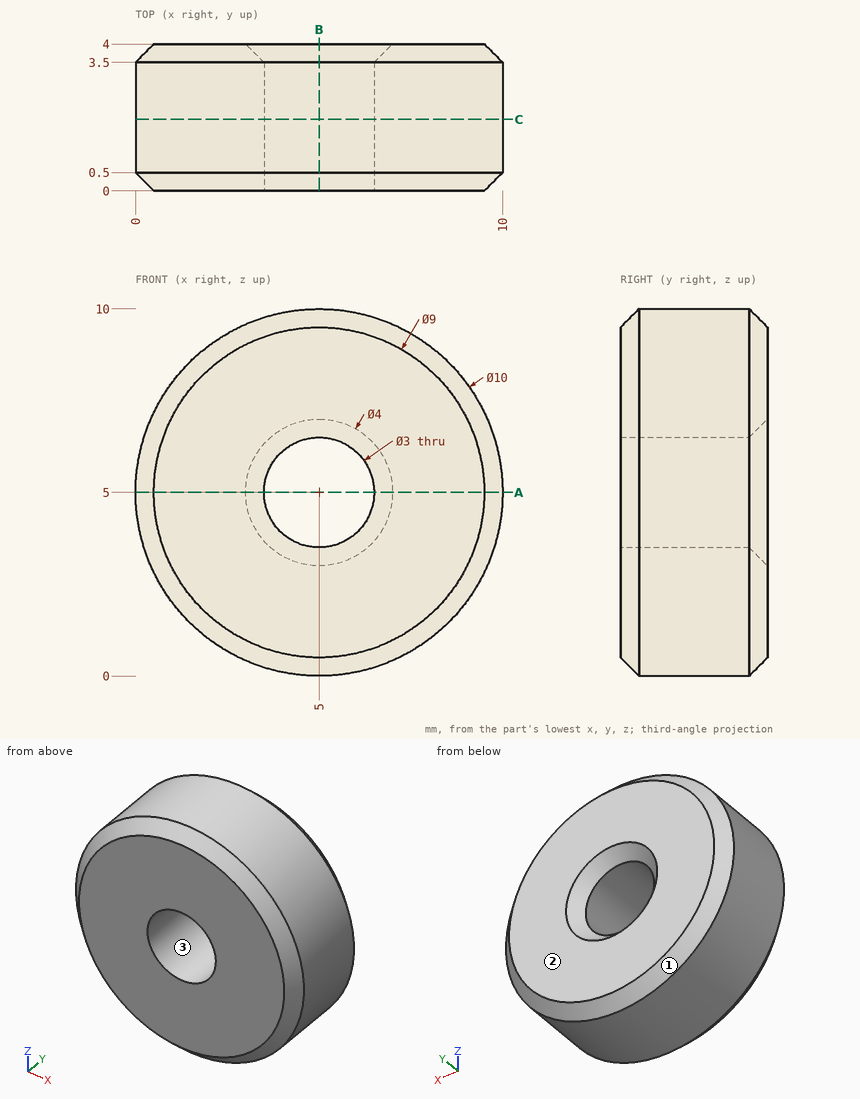
The figure shows three views and two pictorial views of one solid part (mm, origin at its lowest corner). Answer the questions. Round coordinates to 2 decimals unless told otherwise and drop trailing zeros. Loops run counter-clockwise (first coordinate to the right, second up) from the corner with the lowest first, then second, coordinate; pieces in that order, holes last. Notation, with made-up numbers: M -2,20 L 11,20 A16 ccw 11,45 Z; hole C -0.5,23 d10. An arc over 180 degrees is marked long. Write each question's results on one line, items separated by ' | '. Start each with the question number.
1) Straight lines are drawn through the part: probe 1 along X at (y, z) = (0.8, 5); probe 2 along Z at (x, y) = (6, 0.4); probe 3 along X at (y, z) = (1.1, 6). For each, find the intervals that lie inside material, in ascending order.
2) Determine the mould class of the marked faces 1, 2 and 3 for opening direction X: pulls with the +X half, pulls with the -X half, needs draft (parallel to the pull), parting line crosses it, or undercut.
3) Find section B-B on x = 5. Write down the section's boundary in (y, z), plus the area to 4 significant figures.
4) Each of these flat-tipped pins is pushed along its axis until it touches: pin 1 (1 mm diameter, centred on y = 1, z = 1.5, fed in from -X); pin 2 (1 mm diameter, centred on y = 2.5, z = 4, fed in from -X). Where does it stop, or does it pass through?
5) Find section C-C on y = 1.95. Write down the section's boundary in (x, z), plus the area to 3 significant figures.
6) Find section A-A on z = 5. Write down the section's boundary in (x, y).
Final values:
1) probe 1: 0 to 3.5, 6.5 to 10 | probe 2: 0.2 to 3.88, 6.12 to 9.8 | probe 3: 0.1 to 3.88, 6.12 to 9.9
2) face 1: parting line crosses it | face 2: needs draft | face 3: undercut
3) outline: M 0,0.5 L 0.5,0 L 3.5,0 L 4,0.5 L 4,3 L 3.5,3.5 L 0,3.5 Z; M 0,6.5 L 3.5,6.5 L 4,7 L 4,9.5 L 3.5,10 L 0.5,10 L 0,9.5 Z | area: 27.25 mm²
4) pin 1: x = 1 | pin 2: x = 0.03
5) outline: C 5,5 d10; hole C 5,5 d3 | area: 71.5 mm²
6) outline: M 0,0.5 L 0.5,0 L 3.5,0 L 3.5,3.5 L 3,4 L 0.5,4 L 0,3.5 Z; M 6.5,0 L 9.5,0 L 10,0.5 L 10,3.5 L 9.5,4 L 7,4 L 6.5,3.5 Z
